Read the model definition and answer for the solid it produces. Units are mm, in the model's axes. A direction names the side the tool comes from. Coordinates: 2 decimals unless noted, no trailing zeros. Order: outer loops, then holes, each group sorted by start corner. A loop starts at its lowest first (then second) coordinate and runs counter-clockwise, first axis right, second up. Notation, with made-up numbers: M -37,34 L -18,34 A33 ccw -18,70 Z; hole C 31,-24 d5. An arc over 180 degrees is marked long. Write each question's results on one line, items separated by ' | '.
```python
from build123d import *

# Parameters (mm, degrees)
BOSS_EXTRUDE1_DEPTH = 2.5
SKETCH2_R           = 1.7
CUT_EXTRUDE1_DEPTH  = 1.5
FILLET1_R           = 1.5


with BuildPart() as part:
    # Sketch1 → Boss-Extrude1 (new body)
    with BuildSketch(Plane.XY):
        Polygon((-6.06419618, 12.7), (-6.06419618, 9.2), (1.63580382, 0), (5.44580382, 0), (5.44580382, 12.7), align=None)
    extrude(amount=BOSS_EXTRUDE1_DEPTH)

    # Sketch2 → Cut-Extrude1 (cut)
    with BuildSketch(Plane.XY.offset(2.5)):
        with Locations((-2.81419618, 9.2)):
            Circle(SKETCH2_R)
    extrude(amount=-CUT_EXTRUDE1_DEPTH, mode=Mode.SUBTRACT)

    # Fillet1
    fillet1_edges = [part.edges().sort_by_distance(p)[0] for p in [
        (3.54080382, 0, 0),
        (-2.21419618, 4.6, 0),
        (-6.06419618, 10.95, 0),
        (-0.30919618, 12.7, 0),
        (-6.06419618, 9.2, 1.25),
        (-6.06419618, 12.7, 1.25),
    ]]
    fillet(fillet1_edges, radius=FILLET1_R)

    # Mirror2: part across plane


with BuildPart() as part_1:
    add(part.part)
    add(part.part.mirror(Plane(origin=(5.44580382, 0, 2.5), x_dir=(0, 0, 1), z_dir=(-1, 0, 0))))


solid = part_1.part
```
(1) Given pin 1 (2 mm diameter, centred on x = -2.81, y = 9.2, fed in from +Z), flat-ended and moving along its own axis, determine where the tip first touches the part or whether it passes through.
Conclusion:
pin 1: z = 1
(2) The part is cut by section C-C, the plane z = 0.6. Write down the section's boundary in (x, y), then the cut area to 3 significant figures.
Conclusion:
outline: M -5.76,9.74 A1.2 ccw -5.48,8.97 L 1.78,0.3 L 9.12,0.3 L 16.38,8.97 A1.2 ccw 16.66,9.74 L 16.66,11.2 A1.2 ccw 15.46,12.4 L -4.56,12.4 A1.2 ccw -5.76,11.2 Z | area: 203 mm²
(3) The part is cut by section B-B, the plane y = 10.5. Write down the section's boundary in (x, z), then the cut area to 3 significant figures.
Conclusion:
outline: M -6.06,1.5 A1.5 ccw -4.56,0 L 15.46,0 A1.5 ccw 16.96,1.5 L 16.96,2.5 L 14.8,2.5 L 14.8,1 L 12.61,1 L 12.61,2.5 L -1.72,2.5 L -1.72,1 L -3.91,1 L -3.91,2.5 L -6.06,2.5 Z | area: 50.0 mm²
(4) Straight lines are drawn through the part: line 1 (Y direction, x = 5.25, z = 1.4); line 2 (Y direction, x = 14, z = 2.05); line 3 (Y direction, x = -2, z = 2). For each, find the intervals that lie inside material, in ascending order.
Conclusion:
line 1: 0 to 12.7 | line 2: 5.67 to 7.53, 10.87 to 12.7 | line 3: 4.34 to 7.71, 10.69 to 12.7
(5) For faces 1 (the flat face through (14, 9, 1)), 2 (the flat face through (-2.09, 4.45, 1.99)), determine the directions among +Z, -Z, +X, -X, +Y, -Y from which every point of the face is accessible in a straight line to the end or side of a thin tool.
Conclusion:
face 1: +Z | face 2: +Z, -Z, -X, -Y
(6) The part is cut by section A-A, the plane z = 2.15. Write down the section's boundary in (x, y), then the cut area to 3 significant figures.
Conclusion:
outline: M -6.06,9.74 A1.5 ccw -5.71,8.78 L 1.64,0 L 9.26,0 L 16.61,8.78 A1.5 ccw 16.96,9.74 L 16.96,11.2 A1.5 ccw 15.46,12.7 L -4.56,12.7 A1.5 ccw -6.06,11.2 Z; hole C -2.81,9.2 d3.4; hole C 13.71,9.2 d3.4 | area: 202 mm²
(7) The mould has two halves that part along X. Classify faces 3 (the cylindrical face through (12.55, 4.6, 0.45)), 4 (the flat face through (6, 8, 2.5)), 5 (the cylindrical face through (-3.036, 10.886, 1.76)): pulls with the +X half, pulls with the -X half, needs draft (parallel to the pull), parting line crosses it, or undercut.
Conclusion:
face 3: pulls with the +X half | face 4: needs draft | face 5: undercut
